The model under review builds one solid part; all positions refer to its coordinate system, in mm. Coordinates: 2 decimals unless noted, no trailing zeros. Write each loop counter-clockwise with the first axis right and the second up, starting at its lowest first coordinate (ties: lowest second). Pieces come first, ordered by that corner, then holes.
1) For line 1 (Y direction, x = 75, z = 0.4); line 2 (X direction, y = 33.5, z = 0.3); line 3 (X direction, y = -13.5, z = 0.75), list the stretches that pass through material, from the lowest coordinate up.
2) Add section B-B, the plane x = 60. State the section outline as (y, z) points.
3) Mouldability with a two-part tool opening along Y and no side actions: class faces 1 (the flat face through (-1, 1, 0)), 2 (the cylindrical face through (-62.727, -13.142, 0.493)) as released by +Y, released by -Y, zero draft, split by the parting line, or undercut.
4) Add section C-C, the plane x = -75. State the section outline as (y, z) points.
5) Add section A-A, the plane y = 33.5. State the section outline as (x, z) points, then the cut area to 3 significant figures.
Autodesk Inventor part; units mm, degrees
ref_plane "YZ Plane" through (0, 0, 0) normal (1, 0, 0) x (0, 1, 0)
ref_plane "XZ Plane" through (0, 0, 0) normal (0, 1, 0) x (-1, 0, 0)
ref_plane "XY Plane" through (0, 0, 0) normal (0, 0, 1) x (1, 0, 0)
sketch "スケッチ1" plane through (0, 0, 0) normal (0, 0, 1) x (1, 0, 0)
  line L0 (-80, -38.5) -> (80, -38.5)
  line L1 (80, -38.5) -> (80, 38.5)
  line L2 (80, 38.5) -> (-80, 38.5)
  line L3 (-80, 38.5) -> (-80, -38.5)
  line L4 (-80, -38.5) -> (80, 38.5) construction
  line L5 (80, -38.5) -> (-80, 38.5) construction
  point P0 (0, 0)
  dimension "d0" = 160
  dimension "d1" = 77
extrude "プレート1" add sketch "スケッチ1" along normal blind 1
sketch "スケッチ2" plane through (0, 0, 1) normal (0, 0, 1) x (1, 0, 0)
  line L0 (-80, -38.5) -> (-80, 38.5)
  line L1 (80, -38.5) -> (-80, -38.5)
  line L2 (80, 38.5) -> (80, -38.5)
  line L3 (-80, 38.5) -> (80, 38.5)
  line L4 (75, 33.5) -> (75, -33.5)
  line L5 (75, -33.5) -> (-75, -33.5)
  line L6 (-75, -33.5) -> (-75, 33.5)
  line L7 (-75, 33.5) -> (75, 33.5)
  point P0 (0, 0)
  dimension "d3" = 5
hole "穴1" at (-75, 33.5, 1) at (-75, -33.5, 1) at (75, -33.5, 1) at (75, 33.5, 1) direction (0, 0, -1) diameter 3.4 depth 1
sketch "スケッチ3" plane through (0, 0, 1) normal (0, 0, 1) x (1, 0, 0)
  line L0 (80, -38.5) -> (-80, -38.5)
  point P0 (0, 0)
  point P1 (-60, -13.5)
  point P2 (60, -13.5)
  dimension "d11" = 60
  dimension "d12" = 60
  dimension "d13" = 25
  dimension "d14" = 25
hole "穴2" at (-60, -13.5, 1) at (60, -13.5, 1) direction (0, 0, -1) diameter 5.5 end through all
equation "\"d9\" = Thickness"
equation "\"d20\" = Thickness"
equation "\"d2\" = Thickness"
equation "\"BendRadius\" = Thickness"
equation "\"BendReliefWidth\" = Thickness"
equation "\"BendReliefDepth\" = 0.5 * Thickness"
equation "\"CornerReliefSize\" = 4 * Thickness"
equation "\"MinimumRemnant\" = 2 * Thickness"
equation "\"TransitionRadius\" = BendRadius"
equation "\"JacobiRadiusSize\" = Thickness"
equation "\"GapSize\" = Thickness"
properties part number "plate4" material "CFRP"
Geometry results:
1. line 1: y = -38.5 to -35.2, -31.8 to 31.8, 35.2 to 38.5
1. line 2: x = -80 to -76.7, -73.3 to 73.3, 76.7 to 80
1. line 3: x = -80 to -62.75, -57.25 to 57.25, 62.75 to 80
2. outline: (-38.5, 0) - (-16.25, 0) - (-16.25, 1) - (-38.5, 1) - close; (-10.75, 0) - (38.5, 0) - (38.5, 1) - (-10.75, 1) - close
3. face 1: zero draft
3. face 2: undercut
4. outline: (-38.5, 0) - (-35.2, 0) - (-35.2, 1) - (-38.5, 1) - close; (-31.8, 0) - (31.8, 0) - (31.8, 1) - (-31.8, 1) - close; (35.2, 0) - (38.5, 0) - (38.5, 1) - (35.2, 1) - close
5. outline: (-80, 0) - (-76.7, 0) - (-76.7, 1) - (-80, 1) - close; (-73.3, 0) - (73.3, 0) - (73.3, 1) - (-73.3, 1) - close; (76.7, 0) - (80, 0) - (80, 1) - (76.7, 1) - close
5. area: 153 mm2
